```python
from build123d import *

# Parameters (mm, degrees)
F0_R     = 8.5
F1_DEPTH = 4
F2_R     = 5
F3_DEPTH = 100
F7_DEPTH = 5
F8_R     = 0.5
F9_DEPTH = 110.1


with BuildPart() as f1:
    # F0 (on Top) → F1 (new body)
    with BuildSketch(Plane.XY):
        Circle(F0_R)
    extrude(amount=F1_DEPTH)

    # F2 (on Top) → F3 (join)
    with BuildSketch(Plane.XY):
        Circle(F2_R)
    extrude(amount=F3_DEPTH)

    # F4 (on Right) → F5 (revolve)
    with BuildSketch(Plane.YZ):
        with BuildLine():
            Line((3, 102), (0, 102))
            Line((0, 102), (0, 100))
            Line((0, 100), (5, 100))
            ThreePointArc((5, 100), (3.585786, 100.585786), (3, 102))
        make_face()
    revolve(axis=Axis((0, 0, 101), (0, 0, -1)))

    # F6 (on face) → F7 (join)
    with BuildSketch(Plane.XY.offset(102)):
        Polygon((0.087017, -0.996207), (0.906249, -0.422744), (0.819232, 0.573463), (-0.087017, 0.996207), (-0.906249, 0.422744), (-0.819232, -0.573463), align=None)
    extrude(amount=F7_DEPTH)

    # F8 (on face) → F9 (cut)
    with BuildSketch(Plane.XY.offset(107)):
        Circle(F8_R)
    extrude(amount=-F9_DEPTH, mode=Mode.SUBTRACT)


solid = f1.part
```
Check sheet for the modelled part. Datum: model origin and axes. Units: mm. A direction names the side the tool comes from. Round coordinates to 2 decimals unless told otherwise and drop trailing zeros. Loops run counter-clockwise (first coordinate to the right, second up) from the corner with the lowest first, then second, coordinate; pieces in that order, holes last. Notation, with made-up numbers: (-33, 14) -> (20, 14) arc R25 ccw to (20, 43) -> close; hole circle Ø9 at (26.25, -40). An arc over 180 degrees is marked (long way). Answer in a Markdown table with one row per item.
Q1. Set-up check for faces 1 (the face through (4.57, 7.167, 1.972)), 2 (the face through (-1, 1, 102)): record each of +Z, -Z, +X, -X, +Y, -Y from which the full face is reachable in a straight line by a thin tool's end or side.
Data:
| item | result |
|---|---|
| face 1 | +Z, -Z |
| face 2 | +Z |
Q2. Go/stop test with flat-tipped pins: P1, Ø10, axis at x = 4.5, z = 71.5, coming from the -Y side; P2, Ø5, axis at x = 2, y = -0.5, coming from the +Z side; P3, Ø4, axis at y = 3.5, z = 35.5, coming from the -X side; P4, Ø5, axis at x = -3.5, z = 17, coming from the +Y side. Record where each tip stops, or that it passes through.
Data:
| item | result |
|---|---|
| P1 | stops at y = -5 |
| P2 | stops at z = 107 |
| P3 | stops at x = -4.77 |
| P4 | stops at y = 4.9 |
Q3. Thickness scan on L1, parallel to Y at x = 0, z = 79.5; L2, parallel to Z at x = 0.25, y = -1.25; L3, parallel to Y at x = -4, z = 82. Record the ranges inside material, lowest first.
Data:
| item | result |
|---|---|
| L1 | y = -5 to -0.5, 0.5 to 5 |
| L2 | z = 0 to 102 |
| L3 | y = -3 to 3 |
Q4. Sectioned sample at A-A on z = 33. Enter the section's corners in (x, y), then the cut area to 3 significant figures.
Data:
| item | result |
|---|---|
| outline | circle Ø10 at (0, 0); hole circle Ø1 at (0, 0) |
| area | 77.8 mm^2 |
Q5. Sectioned sample at B-B on y = -7. Enter the section's corners in (x, z).
Data:
| item | result |
|---|---|
| outline | (-4.82, 0) -> (4.82, 0) -> (4.82, 4) -> (-4.82, 4) -> close |
